Can you work these out from the model? Positions are in its coordinate system, mm. A direction names the side the tool comes from. Round coordinates to 2 decimals unless told otherwise and drop trailing zeros. Write each loop counter-clockwise with the first axis right and the second up, starting at its lowest first coordinate (ties: lowest second). Pieces come first, ordered by that corner, then holes. Notation, with made-up numbers: (-39.75, 55) - (-11.75, 55) arc R37 cw to (-11.75, 93) - close; hole circle Ø7 at (56, 24.25). An arc over 180 degrees is marked (long way). One line per item, written item: value. Start each with the question number.
(1) I want a section at D-D on y = 5. List the corners of the cut face in (x, z) for me, plus the area to 3 significant figures.
(2) I want a section at C-C on z = 3.05. List the corners of the cut face in (x, y) for me, plus the area to 3 significant figures.
(3) Thinking about a two-plate mould opening in X: for faces 4 (the face through (25, 10, 2)), 5 (the face through (51.86, 0.9, 2.54)), 6 (the face through (55.335, -12.579, 2.535)), 7 (the face through (50, -18, 3)), which applies, +X half, -X half, draft (parallel to the pull), parting line (faces both ways), or undercut?
(4) I'm going to push flat-ended pins straight in: pin 1 Ø1.7 at (x, y) = (6, -23) entering from -Z; pin 2 Ø2 at (y, z) = (5.5, 1.5) entering from +X; pin 3 Ø0.8 at (x, z) = (54.5, 2) entering from +Y. Where does each tip first touch, or does it pass through?
(5) If I drill on L1, parallel to Y at x = 54, z = 2.7; L2, parallel to Y at x = 6, z = 3.25; L3, parallel to X at y = -16.5, z = 4.15, over which ranges is the centre line in solid material (lowest first)? Write a range as from..to.
(6) I want a section at B-B on x = 46. List the corners of the cut face in (y, z) for me.
(7) I want a section at A-A on y = -13. List the corners of the cut face in (x, z) for me.
(8) On a 3-axis mill with a long thin cutter (end or side, diameter ignored), from which of +Z, -Z, +X, -X, +Y, -Y can I reach the whole of each face in a straight line? I mean faces 1 (the face through (0.86, 9.1, 2.54)), 2 (the face through (10, -18, 3)), 3 (the face through (51, 5, 2)). Say none if no direction works.
from build123d import *

# Parameters (mm, degrees)
SKETCH1_W           = 51
SKETCH1_H           = 10
SKETCH1_R           = 2.55
BOSS_EXTRUDE1_DEPTH = 5
SKETCH2_R           = 1.4
BOSS_EXTRUDE2_DEPTH = 5
FILLET1_R           = 3


with BuildPart() as part:
    # Sketch1 → Boss-Extrude1 (new body)
    with BuildSketch(Plane.XY):
        with Locations((25.5, 5)):
            Rectangle(SKETCH1_W, SKETCH1_H)
        with Locations((5, 5)):
            Circle(SKETCH1_R, mode=Mode.SUBTRACT)
        with Locations((46, 5)):
            Circle(SKETCH1_R, mode=Mode.SUBTRACT)
    extrude(amount=BOSS_EXTRUDE1_DEPTH)

    # Sketch2 → Boss-Extrude2 (add)
    with BuildSketch(Plane.XY.offset(5)):
        Polygon((10, -28), (10, -8), (50, -8), (50, -28), (58, -28), (58, 0), (51, 0), (0, 0), (0, -28), align=None)
        with Locations((6, -23)):
            Circle(SKETCH2_R, mode=Mode.SUBTRACT)
        with Locations((6, -13)):
            Circle(SKETCH2_R, mode=Mode.SUBTRACT)
        with Locations((54, -23)):
            Circle(SKETCH2_R, mode=Mode.SUBTRACT)
        with Locations((54, -13)):
            Circle(SKETCH2_R, mode=Mode.SUBTRACT)
    extrude(amount=-BOSS_EXTRUDE2_DEPTH)

    # Fillet1
    fillet1_edges = [part.edges().sort_by_distance(p)[0] for p in [
        (0, -28, 2.5),
        (58, 0, 2.5),
        (58, -28, 2.5),
        (0, 10, 2.5),
        (51, 10, 2.5),
        (51, 0, 2.5),
    ]]
    fillet(fillet1_edges, radius=FILLET1_R)


solid = part.part
Established:
1. outline: (0, 0) - (2.45, 0) - (2.45, 5) - (0, 5) - close; (7.55, 0) - (43.45, 0) - (43.45, 5) - (7.55, 5) - close; (48.55, 0) - (51, 0) - (51, 5) - (48.55, 5) - close
1. area: 204 mm2
2. outline: (0, -25) arc R3 ccw to (3, -28) - (10, -28) - (10, -8) - (50, -8) - (50, -28) - (55, -28) arc R3 ccw to (58, -25) - (58, -3) arc R3 ccw to (55, 0) - (54, 0) arc R3 cw to (51, 3) - (51, 7) arc R3 ccw to (48, 10) - (3, 10) arc R3 ccw to (0, 7) - close; hole circle Ø5.1 at (5, 5); hole circle Ø2.8 at (6, -23); hole circle Ø2.8 at (6, -13); hole circle Ø5.1 at (46, 5); hole circle Ø2.8 at (54, -23); hole circle Ø2.8 at (54, -13)
2. area: 1,260 mm2
3. face 4: draft
3. face 5: +X half
3. face 6: undercut
3. face 7: undercut
4. pin 1: through
4. pin 2: x = 51
4. pin 3: y = 0
5. L1: -28..-24.4, -21.6..-14.4, -11.6..0
5. L2: -28..-24.4, -21.6..-14.4, -11.6..2.65, 7.35..10
5. L3: 0..10, 50..58
6. outline: (-8, 0) - (2.45, 0) - (2.45, 5) - (-8, 5) - close; (7.55, 0) - (10, 0) - (10, 5) - (7.55, 5) - close
7. outline: (0, 0) - (4.6, 0) - (4.6, 5) - (0, 5) - close; (7.4, 0) - (10, 0) - (10, 5) - (7.4, 5) - close; (50, 0) - (52.6, 0) - (52.6, 5) - (50, 5) - close; (55.4, 0) - (58, 0) - (58, 5) - (55.4, 5) - close
8. face 1: +Z, -Z, -X, +Y
8. face 2: +Z, -Z, -Y
8. face 3: +Z, -Z, +X, +Y
